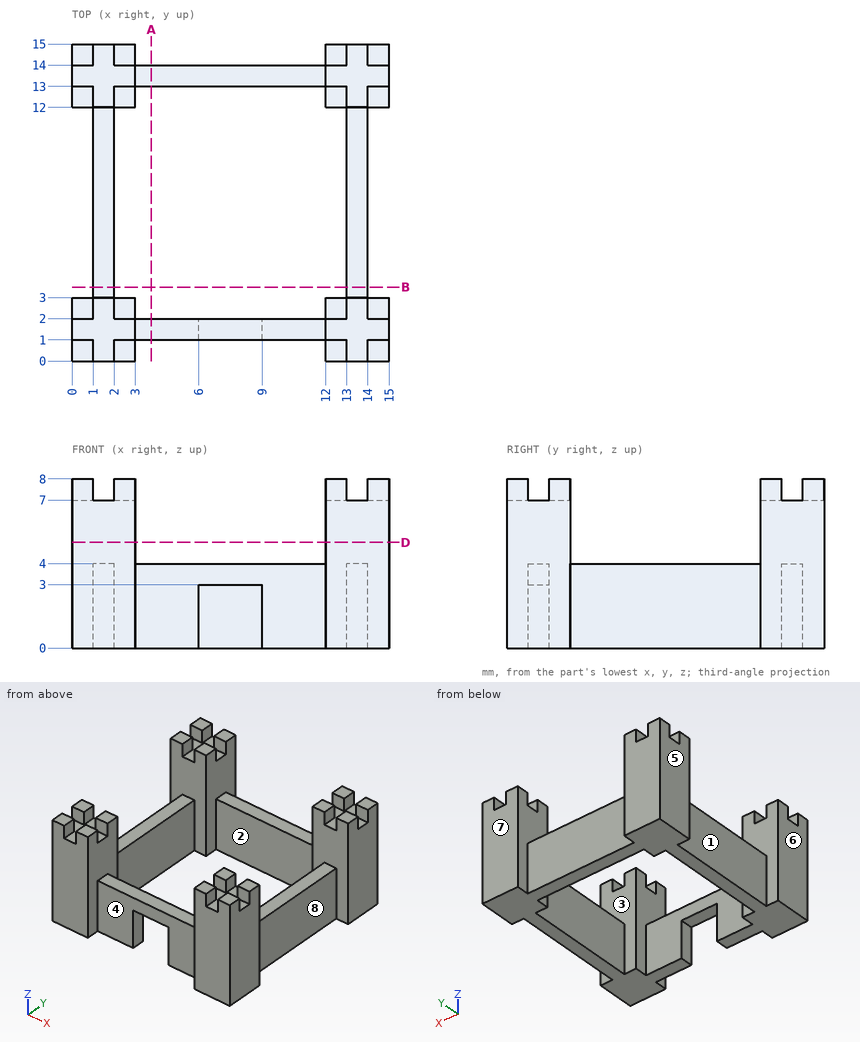
Geometry check sheet. Reference: drawing and pictorial views, mm from the part's lowest x, y, z. A direction names the side the tool comes from. Coordinates: 2 decimals unless noted, no trailing zeros. Order: outer loops, then holes, each group sorted by start corner. A loop starts at its lowest first (then second) coordinate and runs counter-clockwise, first axis right, second up. Notation, with made-up numbers: (-11.5, -37) -> (31.5, -37) arc R14 cw to (31.5, -32) -> close; hole circle Ø5 at (75.25, 5.25). An arc over 180 degrees is marked (long way). Put each result on its own line as item: value. Start each with the question number.
1) Go/stop test with flat-tipped pins: pin 1 (2 mm diameter, centred on x = 8, z = 1.5, fed in from +Y); pin 2 (1.5 mm diameter, centred on x = 6.5, y = 4.5, fed in from +Z); pin 3 (0.5 mm diameter, centred on x = 9, y = 13.5, fed in from +Z); pin 4 (2 mm diameter, centred on y = 8.5, z = 1.5, fed in from -X). Record where each tip stops, or that it passes through.
2) Material ranges on L1, parallel to X at y = 14.25, z = 7.75; L2, parallel to X at y = 13, z = 6, recorded low to high.
3) Cross-section at A-A (x = 3.75). Enter the section's corners in (y, z), plus the area to 3 significant figures.
4) Cross-section at D-D (z = 5). Enter the section's corners in (x, y).
5) Tool access check on the marked faces 1, 2, 3, 4 and 5. Record the directions out of +Z, -Z, +X, -X, +Y, -Y that give a thin tool (end or side, any length) a straight path to the whole face; none if there is none.
6) Release check for a two-part mould opening along Y. For the marked faces 6, 7 and 8 record: pulls with the +Y half, pulls with the -Y half, needs draft (parallel to the pull), parting line crosses it, or undercut.
Geometry check:
1. pin 1: stops at y = 14
1. pin 2: passes through
1. pin 3: stops at z = 4
1. pin 4: stops at x = 1
2. L1: x = 0 to 1, 2 to 3, 12 to 13, 14 to 15
2. L2: x = 0 to 3, 12 to 15
3. outline: (1, 0) -> (2, 0) -> (2, 4) -> (1, 4) -> close; (13, 0) -> (14, 0) -> (14, 4) -> (13, 4) -> close
3. area: 8.00 mm^2
4. outline: (0, 0) -> (3, 0) -> (3, 3) -> (0, 3) -> close; (0, 12) -> (3, 12) -> (3, 15) -> (0, 15) -> close; (12, 0) -> (15, 0) -> (15, 3) -> (12, 3) -> close; (12, 12) -> (15, 12) -> (15, 15) -> (12, 15) -> close
5. face 1: +Z, -Z, -X
5. face 2: +Z, -Z
5. face 3: +Z
5. face 4: +Z, -Z, -Y
5. face 5: +Z, -Z, -X, +Y, -Y
6. face 6: needs draft
6. face 7: pulls with the +Y half
6. face 8: undercut
